Read the model definition and answer for the solid it produces. Units are mm, in the model's axes. Face numbers are marked on the shaded views. A direction names the side the tool comes from. Round coordinates to 2 decimals unless told otherwise and drop trailing zeros. Loops run counter-clockwise (first coordinate to the right, second up) from the corner with the lowest first, then second, coordinate; pieces in that order, holes last. Notation, with made-up numbers: (26.25, 19.5) - (50.25, 19.5) arc R5 ccw to (50.25, 24.5) - close; hole circle Ø9 at (54.5, -39.75). An arc over 180 degrees is marked (long way). Use CSV: the item, a comma, the result in double quotes. Start each with the question number.
1. Find section C-C (y = 3). Give the vertices of the cut face in (x, z).
2. Find section D-D (z = -41.5). Give the vertices of the cut face in (x, y), and give its area (3 significant figures).
3. A tool of negligible diameter and unlimited length cuts with its end or side. For the marked faces 5, 6, 7 and 8, from which of +Z, -Z, +X, -X, +Y, -Y can it reach the whole face along a straight path? Write none if from no direction.
4. Determine the mould class of the marked faces 1, 2, 3 and 4 for opening direction X: +X half, -X half, draft (parallel to the pull), parting line (faces both ways), or undercut.
5. Find section A-A (z = -25). Give the vertices of the cut face in (x, y), and give its area (3 significant figures).
6. Find section B-B (x = 31.75). Give the vertices of the cut face in (y, z).
7. Given pin 1 Ø6 at (x, y) = (29, 8) entering from -Z; pin 2 Ø5 at (x, y) = (19.5, 4.5) entering from +Z; pin 3 Ø10 at (x, z) = (69.5, -23) entering from +Y, each flat-ended and moving along its own axis, determine where each tip first touches the part or whether it passes through.
8. Consider line 1 along X through (y, z) = (3.25, -9.5); line 2 along Z through (x, y) = (76, 8.25); line 3 along Z through (x, y) = (69.68, 16.25). Determine where each line is inside the solid, lowest interval first.
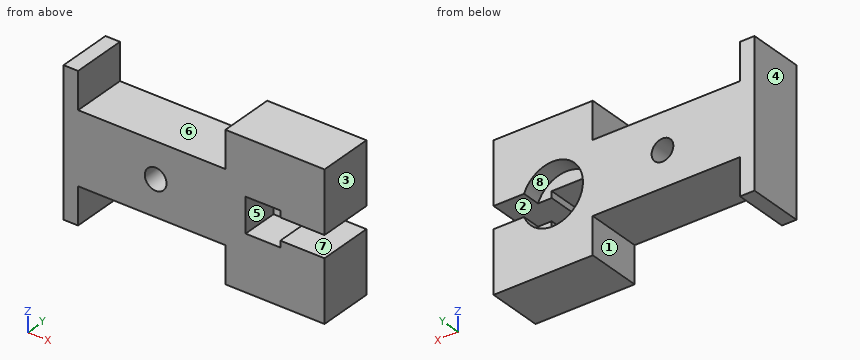
Autodesk Inventor part; units mm, degrees
ref_plane "YZ Plane" through (0, 0, 0) normal (1, 0, 0) x (0, 1, 0)
ref_plane "XZ Plane" through (0, 0, 0) normal (0, 1, 0) x (-1, 0, 0)
ref_plane "XY Plane" through (0, 0, 0) normal (0, 0, 1) x (1, 0, 0)
sketch "Sketch1" plane through (0, 0, 0) normal (0, 1, 0) x (-1, 0, 0)
  line L0 (0, 0) -> (-90, 0)
  line L1 (-90, 0) -> (-90, -50)
  line L2 (-90, -50) -> (0, -50)
  line L3 (0, -50) -> (0, 0)
  line L4 (0, 0) -> (-5, 0)
  line L5 (0, -50) -> (-5, -50)
  line L6 (-5, -50) -> (-5, -37.3)
  line L7 (-5, 0) -> (-5, -12.7)
  line L8 (-5, -12.7) -> (-55.8, -12.7)
  line L9 (-55.8, -12.7) -> (-55.8, 0)
  line L10 (-55.8, 0) -> (-5, 0)
  line L11 (-5, 0) -> (-5, -12.7)
  line L12 (-5, -37.3) -> (-55.8, -37.3)
  line L13 (-55.8, -37.3) -> (-55.8, -50)
  line L14 (-55.8, -50) -> (-5, -50)
  line L15 (-5, -50) -> (-5, -37.3)
  dimension "d0" = 90
  dimension "d1" = 50
  dimension "d4" = 5
  dimension "d5" = 5
  dimension "d6" = 12.7
  dimension "d7" = 12.7
  dimension "d8" = 50.8
  dimension "d9" = 12.7
  dimension "d10" = 50.8
  dimension "d11" = 12.7
extrude "Extrusion2" add sketch "Sketch1" along normal blind 19.05 contours L3 L2 L6 L12 L13 L1 L0 L9 L8 L7
sketch "Sketch3" plane through (0, 19.05, 0) normal (0, 1, 0) x (1, 0, 0)
  line L0 (90, 0) -> (90, 50)
  line L1 (90, 25) -> (74.76, 25)
  line L2 (90, 25) -> (90, 28.75)
  line L3 (90, 25) -> (90, 21.2408)
  line L4 (90, 21.2408) -> (74.76, 21.2408)
  line L5 (74.76, 21.2408) -> (74.76, 28.7408)
  line L6 (74.76, 28.7408) -> (90, 28.7408)
  line L7 (90, 28.7408) -> (90, 21.2408)
  point P0 (0, 0)
  dimension "d18" = 15.24
  dimension "d19" = 3.75
  dimension "d20" = 3.7592
  dimension "d21" = 15.24
  dimension "d22" = 7.5
extrude "Extrusion4" cut sketch "Sketch3" against normal blind 19.05
sketch "Sketch4" plane through (0, 19.05, 0) normal (0, 1, 0) x (1, 0, 0)
  line L0 (74.76, 28.7408) -> (74.76, 21.2408)
  line L1 (74.76, 24.9908) -> (74.76, 30.9852)
  line L2 (74.76, 30.9852) -> (62.76, 30.9852)
  line L3 (62.76, 30.9852) -> (62.76, 18.9964)
  line L4 (62.76, 18.9964) -> (74.76, 18.9964)
  line L5 (74.76, 18.9964) -> (74.76, 30.9852)
  point P0 (0, 0)
  dimension "d25" = 5.9944
  dimension "d26" = 12
  dimension "d27" = 11.9888
extrude "Extrusion5" cut sketch "Sketch4" against normal blind 19.05
sketch "Sketch5" plane through (0, 19.05, 0) normal (0, 1, 0) x (1, 0, 0)
  circle A0 centre (69.68, 24.9908) radius 10.5
  point P0 (0, 0)
  dimension "d30" = 21
extrude "Extrusion6" cut sketch "Sketch5" against normal blind 6.35
sketch "Sketch6" plane through (0, 19.05, 0) normal (0, 1, 0) x (1, 0, 0)
  line L0 (0, 50) -> (0, 0)
  line L1 (0, 25) -> (31.75, 25)
  circle A0 centre (31.75, 25) radius 3.75
  dimension "d33" = 31.75
  dimension "d34" = 7.5
extrude "Extrusion7" cut sketch "Sketch6" against normal blind 19.05
properties part number "Maglev_holder"
Filled sheet:
1,outline,"(0, -50) - (5, -50) - (5, -37.3) - (55.8, -37.3) - (55.8, -50) - (90, -50) - (90, -28.74) - (74.76, -28.74) - (74.76, -30.99) - (62.76, -30.99) - (62.76, -19) - (74.76, -19) - (74.76, -21.24) - (90, -21.24) - (90, 0) - (55.8, 0) - (55.8, -12.7) - (5, -12.7) - (5, 0) - (0, 0) - close; hole circle Ø7.5 at (31.75, -25)"
2,outline,"(0, 0) - (5, 0) - (5, 19.05) - (0, 19.05) - close; (55.8, 0) - (90, 0) - (90, 19.05) - (55.8, 19.05) - close"
2,area,"747 mm²"
3,face 5,"+Y, -Y"
3,face 6,"+Z, +Y, -Y"
3,face 7,"+X, +Y, -Y"
3,face 8,"+Y"
4,face 1,"undercut"
4,face 2,"draft"
4,face 3,"+X half"
4,face 4,"-X half"
5,outline,"(0, 0) - (28, 0) - (28, 19.05) - (0, 19.05) - close; (35.5, 0) - (62.76, 0) - (62.76, 12.7) - (59.18, 12.7) - (59.18, 19.05) - (35.5, 19.05) - close"
5,area,"1,030 mm²"
6,outline,"(0, -37.3) - (19.05, -37.3) - (19.05, -28.75) - (0, -28.75) - close; (0, -21.25) - (19.05, -21.25) - (19.05, -12.7) - (0, -12.7) - close"
7,pin 1,"stops at z = -37.3"
7,pin 2,"stops at z = -12.7"
7,pin 3,"stops at y = 12.7"
8,line 1,"x = 0 to 5, 55.8 to 90"
8,line 2,"z = -50 to -28.74, -21.24 to 0"
8,line 3,"z = -50 to -35.49, -14.49 to 0"
